from build123d import *

# Parameters (mm, degrees)
F0_W     = 76.2
F0_H     = 95.25
F1_DEPTH = 69.85
F3_DEPTH = 51.308
F4_W     = 44.45
F4_H     = 50.789239
F4_H_2   = 3.390253
F4_W_2   = 28.497008
F5_DEPTH = 133.35
F6_R     = 4.699
F7_DEPTH = 164.846


with BuildPart() as f1:
    # F0 (on Top) → F1 (new body)
    with BuildSketch(Plane.XY):
        with Locations((9.872094, 1.178516)):
            Rectangle(F0_W, F0_H)
    extrude(amount=F1_DEPTH)

    # F2 (on Front) → F3 (cut, symmetric)
    with BuildSketch(Plane.XZ):
        Polygon((23.562269, 41.361105), (23.562269, 69.936105), (-4.496123, 70.178263), (-4.496123, 41.603263), align=None)
    extrude(amount=F3_DEPTH, both=True, mode=Mode.SUBTRACT)

    # F4 (on Right) → F5 (cut, symmetric)
    with BuildSketch(Plane.YZ):
        with Locations((-24.730019, 44.444619)):
            Rectangle(F4_W, F4_H)
        Polygon((-52.010767, 19.05), (-46.955019, 19.05), (-46.955019, 69.839239), (-46.955019, 73.229492), (-52.010767, 73.229492), align=None)
        with Locations((-24.730019, 71.534365)):
            Rectangle(F4_W, F4_H_2)
        Polygon((51.391989, 69.839239), (22.894981, 69.839239), (22.894981, 19.05), (48.294981, 19.05), (51.391989, 19.05), align=None)
        with Locations((37.143485, 71.534365)):
            Rectangle(F4_W_2, F4_H_2)
    extrude(amount=F5_DEPTH, both=True, mode=Mode.SUBTRACT)

    # F6 (on Top) → F7 (cut)
    with BuildSketch(Plane.XY):
        with Locations((-15.527906, 36.103516)):
            Circle(F6_R)
        with Locations((35.272094, 36.103516)):
            Circle(F6_R)
        with Locations((-15.527906, -33.746484)):
            Circle(F6_R)
        with Locations((35.272094, -33.746484)):
            Circle(F6_R)
    extrude(amount=F7_DEPTH, mode=Mode.SUBTRACT)


solid = f1.part
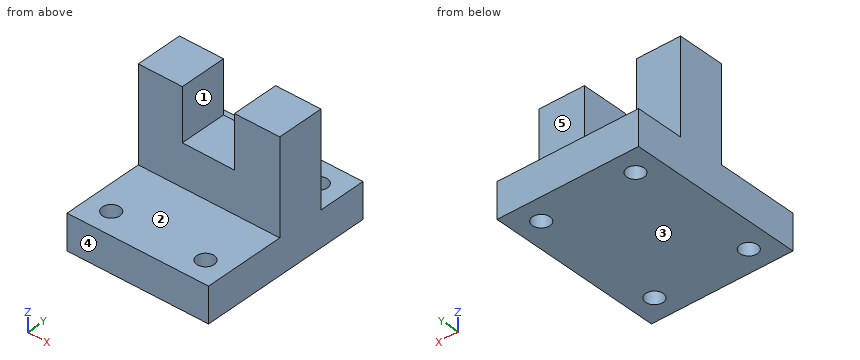
Could you check a few things on this model? Use its own coordinates, in mm. Face numbers are marked on the shaded views. A direction names the side the tool comes from. Give positions to 0.01 mm unless a question says otherwise; leave off trailing zeros. Write each loop counter-clockwise with the first axis right and the second up, starting at its lowest first coordinate (ties: lowest second). Pieces come first, ordered by that corner, then holes. Notation, with made-up numbers: (0, -40) - (41, -40) arc R16 ccw to (41, -10) - close; hole circle Ø10 at (-39.5, 10). An arc over 180 degrees is marked (long way). Use CSV: the item, a comma, the result in double quotes. Start each with the question number.
Item 1: I want a section at C-C, the plane y = 10.5. Please give me the cut outline in (x, z).
Item 2: For the marked faces 1, 2, 3, 4 and 5, which set-ups out of +Z, -Z, +X, -X, +Y, -Y let a thin tool reach every point of the face, with its end or its side?
Item 3: I want a section at A-A, the plane z = 61. Please give me the cut outline in (x, y), then the cut area to 3 significant figures.
Item 4: I want a section at D-D, the plane x = 32.5. Please give me the cut outline in (y, z).
Item 5: I'm going to push flat-ended pins straight in: pin 1 (1 mm diameter, centred on x = 25, z = 59, fed in from -Y) (3 decimals); pin 2 (20.5 mm diameter, centred on x = -3.5, y = 40.5, fed in from +Z); pin 3 (13 mm diameter, centred on x = 28, y = -33, fed in from +Z). Where does each tip first touch, or does it pass through?
Item 6: I want a section at B-B, the plane x = -8.5. Please give me the cut outline in (y, z).
Item 7: If I drill on line 1 along X through (y, z) = (20.5, 64); line 2 along Z through (x, y) = (-6.5, 35.5); line 3 along Y through (x, z) = (31, 31), over which ranges is the centre line in solid material (lowest first)?
Findings:
1,outline,"(-28.23, 0) - (47.97, 0) - (47.97, 69.85) - (23.56, 69.85) - (23.56, 41.36) - (-4.5, 41.6) - (-4.5, 69.85) - (-28.23, 69.85) - close"
2,face 1,"+Z, +Y, -Y"
2,face 2,"+Z, +X, -X, -Y"
2,face 3,"-Z, +X, -X, +Y, -Y"
2,face 4,"+Z, -Z, +X, -X, -Y"
2,face 5,"+Z, +X, -X, +Y"
3,outline,"(-28.23, -2.51) - (-4.5, -2.51) - (-4.5, 22.89) - (-28.23, 22.89) - close; (23.56, -2.51) - (47.97, -2.51) - (47.97, 22.89) - (23.56, 22.89) - close"
3,area,"1,220 mm2"
4,outline,"(-46.45, 0) - (-37.54, 0) - (-37.54, 19.05) - (-46.45, 19.05) - close; (-29.95, 0) - (32.31, 0) - (32.31, 19.05) - (22.89, 19.05) - (22.89, 69.85) - (-2.51, 69.85) - (-2.51, 19.05) - (-29.95, 19.05) - close; (39.9, 0) - (48.8, 0) - (48.8, 19.05) - (39.9, 19.05) - close"
5,pin 1,"stops at y = -2.505"
5,pin 2,"stops at z = 19.05"
5,pin 3,"stops at z = 19.05"
6,outline,"(-46.45, 0) - (48.8, 0) - (48.8, 19.05) - (22.89, 19.05) - (22.89, 69.85) - (-2.51, 69.85) - (-2.51, 19.05) - (-46.45, 19.05) - close"
7,line 1,"x = -28.23 to -4.5, 23.56 to 47.97"
7,line 2,"z = 0 to 19.05"
7,line 3,"y = -2.51 to 22.89"
